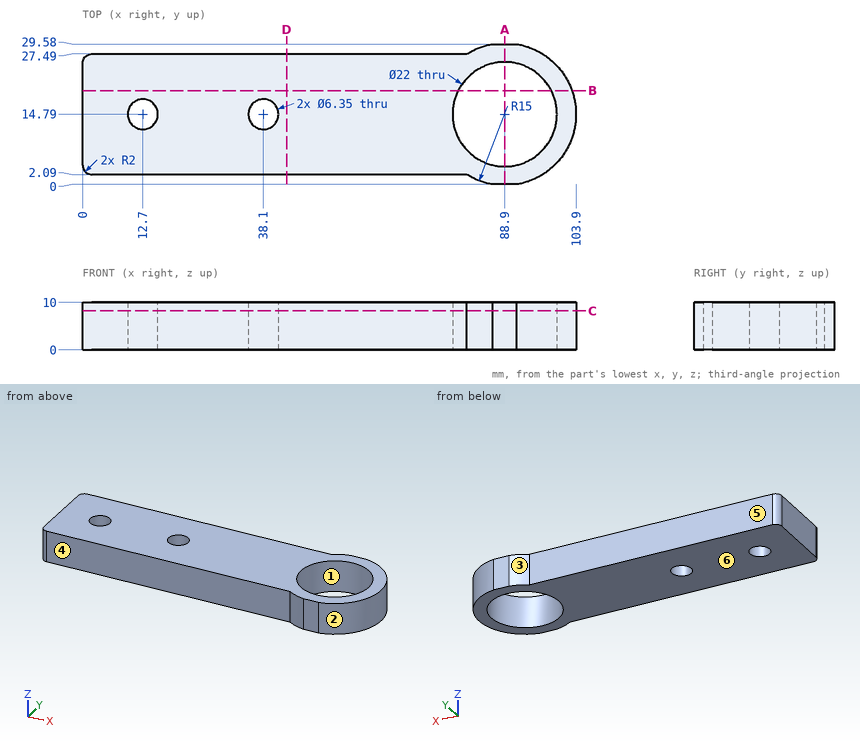
The drawing under review shows one solid part. Ordinate dimensions are in mm from its lowest x, y, z. A direction names the side the tool comes from. Coordinates: 2 decimals unless noted, no trailing zeros. Write each loop counter-clockwise with the first axis right and the second up, starting at its lowest first coordinate (ties: lowest second). Pieces come first, ordered by that corner, then holes. Notation, with made-up numbers: (40.25, -5.5) - (95.25, -5.5) arc R17 ccw to (95.25, -0.5) - close; hole circle Ø10 at (-39, -36.5). An arc over 180 degrees is marked (long way). Answer in a Markdown table with one row per item. Add a question column.
Q1. For probe 1 along X at (y, z) = (14.5, 6.75); probe 2 along Y at (x, z) = (12.7, 7) (1 decimal); probe 3 along Y at (x, z) = (88.9, 7.25), list the stretches that pass through material, from the lowest coordinate up.
Q2. Tool access review of the marked faces 4, 5 and 6: name each direction out of +Z, -Z, +X, -X, +Y, -Y from which nothing blocks a thin tool from reaching the whole face with its end or side.
Q3. We need section C-C, the plane z = 8.25. Count the separate pieces of the cut face and the enclosed holes in it, and give its area (3 significant figures).
Q4. Draft analysis for pull direction Y (two halves, no side actions). For the marked faces 1, 2 and 3, state which applies: +Y half, -Y half, draft (parallel to the pull), parting line (faces both ways), or undercut.
Q5. We need section D-D, the plane x = 43. State the section outline as (y, z) points.
Q6. We need section A-A, the plane x = 88.9. State the section outline as (y, z) points.
Q7. For P1, Ø6, axis at x = 61.5, z = 7.5, coming from the -Y side; P2, Ø7.5, axis at x = 38.1, y = 14.79, coming from the -Z side; P3, Ø3, axis at y = 9.5, z = 2.5, coming from the +X side; P4, Ø3, axis at x = 34.5, z = 5.5, coming from the +Y side, all flat-tipped, find the tip position at first contact; note any pin that passes through.
Q8. We need section B-B, the plane y = 19.75. State the section outline as (x, z) points.
Answer list:
| question | item | result |
|---|---|---|
| 1 | probe 1 | x = 0 to 9.54, 15.86 to 34.94, 41.26 to 77.9, 99.9 to 103.9 |
| 1 | probe 2 | y = 2.1 to 11.6, 18 to 27.5 |
| 1 | probe 3 | y = 0 to 3.79, 25.79 to 29.58 |
| 2 | face 4 | +Z, -Z, -X, -Y |
| 2 | face 5 | +Z, -Z, -X, +Y |
| 2 | face 6 | -Z, +X, -X, +Y, -Y |
| 3 | separate pieces | 1 |
| 3 | enclosed holes | 3 |
| 3 | area | 2,190 mm2 |
| 4 | face 1 | undercut |
| 4 | face 2 | parting line |
| 4 | face 3 | +Y half |
| 5 | outline | (2.09, 0) - (27.49, 0) - (27.49, 10) - (2.09, 10) - close |
| 6 | outline | (0, 0) - (3.79, 0) - (3.79, 10) - (0, 10) - close; (25.79, 0) - (29.58, 0) - (29.58, 10) - (25.79, 10) - close |
| 7 | P1 | stops at y = 2.09 |
| 7 | P2 | stops at z = 0 |
| 7 | P3 | stops at x = 103.41 |
| 7 | P4 | stops at y = 27.49 |
| 8 | outline | (0, 0) - (79.08, 0) - (79.08, 10) - (0, 10) - close; (98.72, 0) - (103.06, 0) - (103.06, 10) - (98.72, 10) - close |
